Design review of the part built by this model. Coordinates are the model's own, in mm. A direction names the side the tool comes from. Round coordinates to 2 decimals unless told otherwise and drop trailing zeros. Loops run counter-clockwise (first coordinate to the right, second up) from the corner with the lowest first, then second, coordinate; pieces in that order, holes last. Notation, with made-up numbers: (-29.75, 11.25) - (-15.75, 11.25) arc R22 cw to (-15.75, 31.25) - close; hole circle Ø4 at (-12.5, 0). An arc over 180 degrees is marked (long way). Return JSON: item names as keys, results as strings. Group by question number.
(1) Wall thickness on L1, parallel to Y at x = 0, z = -2; L2, parallel to Y at x = 22.5, z = -10.5; L3, parallel to Y at x = -15, z = -4: over which ranges is each line inside the solid? List them lowest first. Write a range as [from, to].
(2) Clearance check with flat-ended pins moving along their axes: pin 1 (2 mm diameter, centred on y = -44, z = 17, fed in from -X); pin 2 (2 mm diameter, centred on y = -10, z = -25.5, fed in from +X); pin 3 (3.5 mm diameter, centred on x = 21, z = -16, fed in from -Y). State where each tip first meets the part, or that it passes through.
(3) We need section A-A, the plane y = -31. Write out the cut boundary in (x, z), and give its area (3 significant figures).
(4) For faces 4 (the flat face through (14, -14, -24)), 5 (the flat face through (-16, -14, -25)), 6 (the cylindrical face through (-8.618, -44.521, -20.784)), 7 (the flat face through (16, -14, -25)), list the 3-axis set-ups (+Z, -Z, +X, -X, +Y, -Y) from which the entire face can be reached by the end or side of a thin tool; tool diameter is ignored.
(5) The part is to be moulded in two halves that separate along Y. For faces 1 (the flat face through (19, -23, 19)), 2 (the flat face through (0, -42, 26)), 3 (the flat face through (13, -45, 0)), say which applies: pulls with the +Y half, pulls with the -Y half, needs draft (parallel to the pull), parting line crosses it, or undercut.
(6) We need section B-B, the plane y = -47.5. Write out the cut boundary in (x, z), and give its area (3 significant figures).
(7) We need section C-C, the plane y = -8.5. Write out the cut boundary in (x, z).
from build123d import *

# Parameters (mm, degrees)
BOSS_EXTRUDE1_DEPTH      = 5
BOSS_EXTRUDE2_DEPTH      = 18
BOSS_EXTRUDE3_DEPTH      = 23
SKETCH4_W                = 32
SKETCH4_H                = 25
SKETCH4_H_2              = 8
BOSS_EXTRUDE4_DEPTH      = 1
CUT_EXTRUDE1_DEPTH       = 73.746133918
CUT_EXTRUDE1_DEPTH_BACK  = 73.746133918
WRAP1_START              = -0.5
WRAP1_DEPTH              = 0.5
SKETCH8_R                = 7.5
SKETCH8_R_2              = 0.5
BOSS_EXTRUDE5_DEPTH      = 10
SKETCH9_R                = 8
CUT_EXTRUDE2_DEPTH       = 80.711981534
M3_CLEARANCE_HOLE1_D     = 3.4
M3_CLEARANCE_HOLE1_DEPTH = 8
M3_CLEARANCE_HOLE1_TIP   = 1.021463052
M3_CLEARANCE_HOLE2_D     = 3.4
M3_CLEARANCE_HOLE2_DEPTH = 8
M3_CLEARANCE_HOLE2_TIP   = 1.021463052
M3_CLEARANCE_HOLE3_D     = 3.4
M3_CLEARANCE_HOLE3_DEPTH = 8
M3_CLEARANCE_HOLE3_TIP   = 1.021463052
M3_CLEARANCE_HOLE4_D     = 3.4
M3_CLEARANCE_HOLE4_DEPTH = 8
M3_CLEARANCE_HOLE4_TIP   = 1.021463052
SKETCH22_R               = 22.5
SKETCH22_R_2             = 21.5
CUT_EXTRUDE3_DEPTH       = 3


# Read off the part's stored shape, not the designer's step: Wrap1
with BuildPart() as part:
    # Sketch1 → Boss-Extrude1 (new body)
    with BuildSketch(Plane(origin=(0, 0, 0), x_dir=(1, 0, 0), z_dir=(0, 1, 0))):
        Polygon((-25, 12.5), (-23.126297114, 23.126297114), (-12.5, 25), (12.5, 25), (23.126297114, 23.126297114), (25, 12.5), (25, -12.5), (23.126297114, -23.126297114), (12.5, -25), (-12.5, -25), (-23.126297114, -23.126297114), (-25, -12.5), align=None)
    extrude(amount=-BOSS_EXTRUDE1_DEPTH)

    # Sketch2 → Boss-Extrude2 (add)
    with BuildSketch(Plane.XZ.offset(5)):
        Polygon((-12.5, 25), (-12.5, 12.5), (-25, 12.5), (-25, -12.5), (-12.5, -12.5), (-12.5, -25), (12.5, -25), (12.5, -12.5), (25, -12.5), (25, 12.5), (12.5, 12.5), (12.5, 25), align=None)
    extrude(amount=BOSS_EXTRUDE2_DEPTH)

    # Sketch3 → Boss-Extrude3 (add)
    with BuildSketch(Plane.XZ.offset(23)):
        Polygon((12.5, 25), (-12.5, 25), (-12.5, 12.5), (-25, 12.5), (-25, -12.5), (-12.5, -12.5), (-12.5, -25), (12.5, -25), (12.5, -12.5), (25, -12.5), (25, 12.5), (12.5, 12.5), align=None)
        Polygon((-25, 12.5), (-23.126297114, 23.126297114), (-12.5, 25), (-12.5, 12.5), align=None)
        Polygon((12.5, 25), (23.126297114, 23.126297114), (25, 12.5), (12.5, 12.5), align=None)
        Polygon((-12.5, -25), (-23.126297114, -23.126297114), (-25, -12.5), (-12.5, -12.5), align=None)
        Polygon((25, -12.5), (23.126297114, -23.126297114), (12.5, -25), (12.5, -12.5), align=None)
    extrude(amount=BOSS_EXTRUDE3_DEPTH)

    # Sketch4 → Boss-Extrude4 (add, symmetric)
    with BuildSketch(Plane(origin=(0, 0, -25), x_dir=(-1, 0, 0), z_dir=(0, 0, -1))):
        with Locations((0, -14)):
            Rectangle(SKETCH4_W, SKETCH4_H)
        with Locations((0, -42)):
            Rectangle(SKETCH4_W, SKETCH4_H_2)
    boss_extrude4 = extrude(amount=BOSS_EXTRUDE4_DEPTH, both=True)

    # Mirror2: Boss-Extrude4 across plane
    add(boss_extrude4.mirror(Plane.XY))

    # Sketch6 → Cut-Extrude1 (cut, two sides: drawn at the far end of the back side and taken through both)
    with BuildSketch(Plane(origin=(25, 0, 0), x_dir=(0, 0, -1), z_dir=(1, 0, 0)).offset(-CUT_EXTRUDE1_DEPTH_BACK)):
        Polygon((5, -45), (-5, -45), (-5.176326981, -46), (5.176326981, -46), align=None)
    extrude(amount=CUT_EXTRUDE1_DEPTH + CUT_EXTRUDE1_DEPTH_BACK, mode=Mode.SUBTRACT)

    # Wrap1 outline → Wrap1 (cut)
    with BuildSketch(Plane(origin=(25, 0, 0), x_dir=(0, 0, -1), z_dir=(1, 0, 0)).offset(WRAP1_START)):
        Polygon((0, -41), (-3, -41), (-3, -42), (0, -42), (0, -43), (3, -41.5), (0, -40), align=None)
    wrap1 = extrude(amount=WRAP1_DEPTH, mode=Mode.SUBTRACT)

    # Mirror3: Wrap1 across plane
    add(wrap1.mirror(Plane(origin=(0, 0, 0), x_dir=(0, 0, 1), z_dir=(1, 0, 0))), mode=Mode.SUBTRACT)

    # Sketch8 → Boss-Extrude5 (add)
    with BuildSketch(Plane.XZ.offset(45)):
        with Locations(Location((0, 0, 0), (0, 0, 43.644116102))):
            Circle(SKETCH8_R)
        with Locations(Location((0, 0, 0), (0, 0, 270))):
            Circle(SKETCH8_R_2, mode=Mode.SUBTRACT)
    extrude(amount=BOSS_EXTRUDE5_DEPTH)

    # Sketch9 → Cut-Extrude2 (cut, through all)
    with BuildSketch(Plane(origin=(0, 0, -26), x_dir=(-1, 0, 0), z_dir=(0, 0, -1))):
        with Locations((0, -14)):
            Circle(SKETCH9_R)
    extrude(amount=-CUT_EXTRUDE2_DEPTH, mode=Mode.SUBTRACT)

    # M3 Clearance Hole1
    with Locations(Plane(origin=(25, 0, 0), x_dir=(0, 0, -1), z_dir=(1, 0, 0))):
        with Locations((10.5, -2), (-10.5, -23)):
            Hole(M3_CLEARANCE_HOLE1_D / 2, depth=M3_CLEARANCE_HOLE1_DEPTH)
            with Locations((0, 0, -(M3_CLEARANCE_HOLE1_DEPTH + M3_CLEARANCE_HOLE1_TIP / 2))):  # 118° drill point
                Cone(0, M3_CLEARANCE_HOLE1_D / 2, M3_CLEARANCE_HOLE1_TIP, mode=Mode.SUBTRACT)

    # M3 Clearance Hole2
    with Locations(Plane.ZY.offset(25)):
        with Locations((10.5, -2), (-10.5, -23)):
            Hole(M3_CLEARANCE_HOLE2_D / 2, depth=M3_CLEARANCE_HOLE2_DEPTH)
            with Locations((0, 0, -(M3_CLEARANCE_HOLE2_DEPTH + M3_CLEARANCE_HOLE2_TIP / 2))):  # 118° drill point
                Cone(0, M3_CLEARANCE_HOLE2_D / 2, M3_CLEARANCE_HOLE2_TIP, mode=Mode.SUBTRACT)

    # M3 Clearance Hole3
    with Locations(Plane(origin=(25, 0, 0), x_dir=(0, 0, -1), z_dir=(1, 0, 0))):
        with Locations((0, -12.5)):
            Hole(M3_CLEARANCE_HOLE3_D / 2, depth=M3_CLEARANCE_HOLE3_DEPTH)
            with Locations((0, 0, -(M3_CLEARANCE_HOLE3_DEPTH + M3_CLEARANCE_HOLE3_TIP / 2))):  # 118° drill point
                Cone(0, M3_CLEARANCE_HOLE3_D / 2, M3_CLEARANCE_HOLE3_TIP, mode=Mode.SUBTRACT)

    # M3 Clearance Hole4
    with Locations(Plane.ZY.offset(25)):
        with Locations((0, -12.5)):
            Hole(M3_CLEARANCE_HOLE4_D / 2, depth=M3_CLEARANCE_HOLE4_DEPTH)
            with Locations((0, 0, -(M3_CLEARANCE_HOLE4_DEPTH + M3_CLEARANCE_HOLE4_TIP / 2))):  # 118° drill point
                Cone(0, M3_CLEARANCE_HOLE4_D / 2, M3_CLEARANCE_HOLE4_TIP, mode=Mode.SUBTRACT)

    # Sketch22 → Cut-Extrude3 (cut)
    with BuildSketch(Plane.XZ.offset(46)):
        with Locations(Location((0, 0, 0), (0, 0, 270))):
            Circle(SKETCH22_R)
        with Locations(Location((0, 0, 0), (0, 0, 270))):
            Circle(SKETCH22_R_2, mode=Mode.SUBTRACT)
    extrude(amount=-CUT_EXTRUDE3_DEPTH, mode=Mode.SUBTRACT)


solid = part.part
Solutions:
{
 "1": {"L1": "[-55, -22], [-6, 0]", "L2": "[-46, -3.7], [-0.3, 0]", "L3": "[-45, 0]"},
 "2": {"pin 1": "x = -24.38", "pin 2": "x = 16", "pin 3": "y = -46"},
 "3": {"outline": "(-25, -12.5) - (-23.13, -23.13) - (-12.5, -25) - (12.5, -25) - (23.13, -23.13) - (25, -12.5) - (25, 12.5) - (23.13, 23.13) - (12.5, 25) - (-12.5, 25) - (-23.13, 23.13) - (-25, 12.5) - close", "area": "2,410 mm^2"},
 "4": {"face 4": "+X", "face 5": "-Z, -X", "face 6": "-Y", "face 7": "-Z, +X"},
 "5": {"face 1": "undercut", "face 2": "needs draft", "face 3": "pulls with the -Y half"},
 "6": {"outline": "circle Ø15 at (0, 0); hole circle Ø1 at (0, 0)", "area": "176 mm^2"},
 "7": {"outline": "(-25, -12.5) - (-12.5, -12.5) - (-12.5, -24) - (-16, -24) - (-16, -26) - (-5.81, -26) - (-5.81, 26) - (-16, 26) - (-16, 24) - (-12.5, 24) - (-12.5, 12.5) - (-25, 12.5) - close; (5.81, -26) - (16, -26) - (16, -24) - (12.5, -24) - (12.5, -12.5) - (25, -12.5) - (25, 12.5) - (12.5, 12.5) - (12.5, 24) - (16, 24) - (16, 26) - (5.81, 26) - close"}
}
